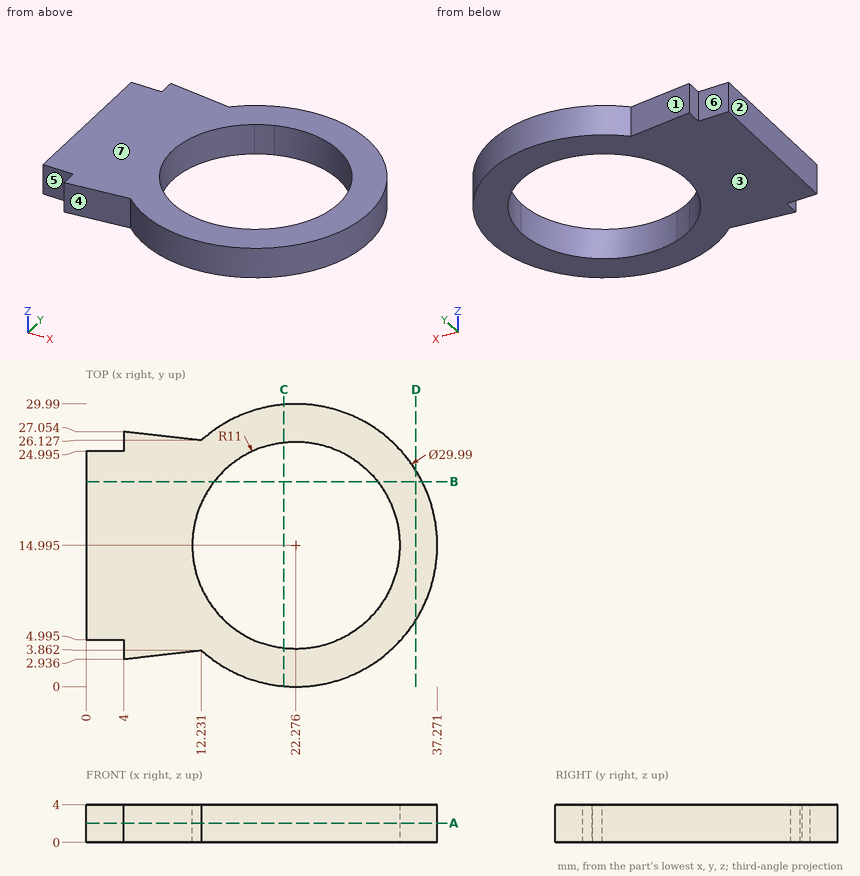
Could you check a few things on this drawing? It's one solid part, dimensions in mm from its lowest x, y, z. A direction names the side the tool comes from. Coordinates: 2 decimals unless noted, no trailing zeros. Loops run counter-clockwise (first coordinate to the right, second up) from the corner with the lowest first, then second, coordinate; pieces in that order, holes last. Notation, with made-up numbers: (44, -30.5) - (90, -30.5) arc R17 cw to (90, -22.5) - close; hole circle Ø4 at (-19, 57.5). An arc over 180 degrees is marked (long way). Return JSON: item names as keys, results as strings. Group by question number.
Item 1: I need wall thicknesses on line 1 (Y direction, x = 30.5, z = 2.4) (1 decimal); line 2 (Y direction, x = 23, z = 2); line 3 (X direction, y = 11.25, z = 1.7) (1 decimal). Which ranges of each line are inside material? Lowest first, please. Write a range as from..to.
Item 2: If we section it at A-A on z = 2.05: Write out the boundary of the cut face in (x, y) (1 decimal).
Item 3: If we section it at B-B on y = 21.75: Write out the boundary of the cut face in (x, z) (1 decimal).
Item 4: If we section it at D-D on x = 35: Write out the boundary of the cut face in (y, z).
Item 5: If we section it at C-C on x = 21: Write out the boundary of the cut face in (y, z) (1 decimal).
Item 6: Will these pins go through, and if not, where does the flat tip stop? P1, Ø1.5, axis at y = 5.5, z = 2, coming from the +X side; P2, Ø0.6, axis at y = 3.5, z = 2, coming from the -X side; P3, Ø5, axis at x = 13, y = 24, coming from the -Z side; P4, Ø2, axis at x = 31, z = 3, coming from the -Y side.
Item 7: We'd pull the mould along X, two halves only. Please class the marked faces 1, 2 and 3: +X half, -X half, draft (parallel to the pull), parting line (faces both ways), or undercut.
Item 8: On a 3-axis mill with a long thin cutter (end or side, diameter ignored), from which of +Z, -Z, +X, -X, +Y, -Y can I reach the whole of each face in a straight line? I mean the marked faces 4, 5, 6 and 7. Say none if no direction works.
Calculated:
{
 "1": {"line 1": "y = 2.5..7.7, 22.3..27.5", "line 2": "y = 0.02..4.02, 25.97..29.97", "line 3": "x = 0..11.9, 32.6..36.8"},
 "2": {"outline": "(0, 5) - (4, 5) - (4, 2.9) - (12.2, 3.9) arc R15 ccw (long way) to (12.2, 26.1) - (4, 27.1) - (4, 25) - (0, 25) - close; hole circle Ø22 at (22.3, 15)"},
 "3": {"outline": "(0, 0) - (13.6, 0) - (13.6, 4) - (0, 4) - close; (31, 0) - (35.7, 0) - (35.7, 4) - (31, 4) - close"},
 "4": {"outline": "(7.06, 0) - (22.93, 0) - (22.93, 4) - (7.06, 4) - close"},
 "5": {"outline": "(0.1, 0) - (4.1, 0) - (4.1, 4) - (0.1, 4) - close; (25.9, 0) - (29.9, 0) - (29.9, 4) - (25.9, 4) - close"},
 "6": {"P1": "stops at x = 34.46", "P2": "stops at x = 4", "P3": "stops at z = 0", "P4": "stops at y = 2.14"},
 "7": {"face 1": "undercut", "face 2": "-X half", "face 3": "draft"},
 "8": {"face 4": "+Z, -Z, -Y", "face 5": "+Z, -Z, -X, -Y", "face 6": "+Z, -Z, -X, +Y", "face 7": "+Z, +X, -X, +Y, -Y"}
}
